```python
from build123d import *

# Parameters (mm, degrees)
SKETCH_1_W          = 3
SKETCH_1_H          = 15
EXTRUDE_1_DEPTH     = 200
EXTRUDE_7_DEPTH     = 3
SKETCH_13_W         = 10.2
SKETCH_13_H         = 3.2
CUT_EXTRUDE_2_DEPTH = 23


with BuildPart() as part:
    # 草图1 → 凸台-拉伸1 (new body)
    with BuildSketch(Plane.XY):
        with Locations((1.5, 7.5)):
            Rectangle(SKETCH_1_W, SKETCH_1_H)
    extrude(amount=EXTRUDE_1_DEPTH)

    # 草图12 → 凸台-拉伸7 (add)
    with BuildSketch(Plane(origin=(0, 9, 0), x_dir=(1, 0, 0), z_dir=(0, 1, 0))):
        Polygon((18, -191.190016229), (23, -105), (23, -95), (18, -8.809983771), (3, -8.809983771), (3, -191.190016229), align=None)
    extrude(amount=-EXTRUDE_7_DEPTH)

    # 草图13 → 切除-拉伸2 (cut)
    with BuildSketch(Plane.XZ.offset(-6)):
        with Locations((14.3, 100)):
            Rectangle(SKETCH_13_W, SKETCH_13_H)
    extrude(amount=-CUT_EXTRUDE_2_DEPTH, mode=Mode.SUBTRACT)


solid = part.part
```
Could you check a few things on this model? Use its own coordinates, in mm. A direction names the side the tool comes from. Coordinates: 2 decimals unless noted, no trailing zeros. Loops run counter-clockwise (first coordinate to the right, second up) from the corner with the lowest first, then second, coordinate; pieces in that order, holes last. Notation, with made-up numbers: M 82.5,89.5 L 113.5,89.5 A21 ccw 113.5,115.5 Z; hole C 32.5,-2 d2. An arc over 180 degrees is marked long. Put each result on its own line as item: value. Start each with the question number.
(1) For faces 1 (the face through (20.535, 7.521, 52.508)), 2 (the face through (8, 6, 99)), 3 (the face through (8, 9, 99)), which set-ups out of +Z, -Z, +X, -X, +Y, -Y let a thin tool reach every point of the face, with its end or its side?
(2) Suppose I cut it at B-B on z = 115.5. Please give me the cut outline in (x, y).
(3) Suppose I cut it at C-C on y = 3.5. Please give me the cut outline in (x, z), then the cut area to 3 significant figures.
(4) I need wall thicknesses on line 1 (Z direction, x = 13.75, y = 6.5); line 2 (Y direction, x = 21.75, z = 96.5); line 3 (X direction, y = 13, z = 43). Which ranges of each line are inside material? Lowest first, please. Write a range as from..to.
(5) Suppose I cut it at D-D on x = 7. Please give me the cut outline in (y, z).
(6) Suppose I cut it at A-A on x = 15.5. Please give me the cut outline in (y, z), then the cut area to 3 significant figures.
(7) Will these pins go through, and if not, where does the flat tip stop? P1, Ø6, axis at x = 17.5, y = 4.5, coming from the -Z side; P2, Ø5, axis at x = 19, y = 12.5, coming from the +Z side; P3, Ø1.5, axis at x = 8.5, z = 170, coming from the +Y side; P4, Ø1.5, axis at x = 7, y = 8, coming from the +Z side.
Solutions:
1. face 1: -Z, +X, +Y, -Y
1. face 2: +Z, -Z, +X, -Y
1. face 3: +Z, -Z, +X, +Y
2. outline: M 0,0 L 3,0 L 3,6 L 22.39,6 L 22.39,9 L 3,9 L 3,15 L 0,15 Z
3. outline: M 0,0 L 3,0 L 3,200 L 0,200 Z
3. area: 600 mm2
4. line 1: z = 8.81..98.4, 101.6..191.19
4. line 2: y = 6..9
4. line 3: x = 0..3
5. outline: M 6,8.81 L 9,8.81 L 9,191.19 L 6,191.19 Z
6. outline: M 6,8.81 L 9,8.81 L 9,98.4 L 6,98.4 Z; M 6,101.6 L 9,101.6 L 9,191.19 L 6,191.19 Z
6. area: 538 mm2
7. P1: stops at z = 8.81
7. P2: passes through
7. P3: stops at y = 9
7. P4: stops at z = 191.19
